Check sheet for the modelled part. Datum: model origin and axes. Units: mm. Face numbers are marked on the shaded views. Round coordinates to 2 decimals unless told otherwise and drop trailing zeros.
Item 1: Go/stop test with flat-tipped pins: pin 1 Ø0.9 at (y, z) = (47.5, 2) entering from -X; pin 2 Ø5.5 at (x, y) = (-15, -38.31) entering from +Z; pin 3 Ø6 at (x, y) = (-57, -19.5) entering from -Z; pin 4 Ø5 at (x, y) = (-17.5, 51.5) entering from +Z. Record where each tip stops, or that it passes through.
Item 2: Cross-section at A-A on y = -38.31. Count the separate pieces of the cut face and the enclosed holes in it, plus the area to 3 significant figures.
Item 3: Release check for a two-part mould opening along X. For the marked faces 1 and 2 record: +X half, -X half, draft (parallel to the pull), parting line (faces both ways), or undercut.
Item 4: Material ranges on line 1 (X direction, y = -38.31, z = 0.65); line 2 (X direction, y = -38.31, z = 0.75); line 3 (X direction, y = 30.5, z = 1.65), recorded low to high.
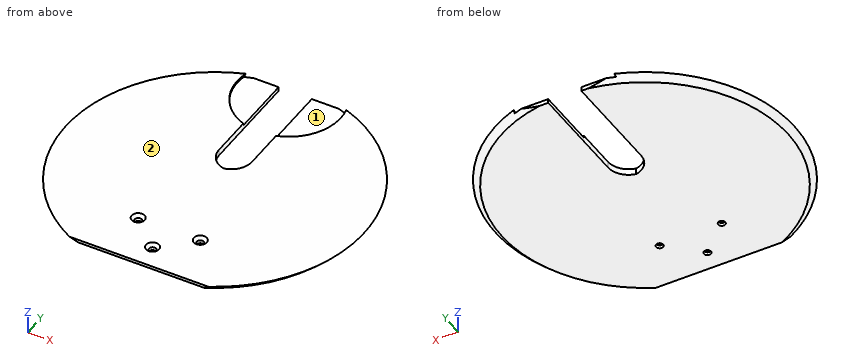
from build123d import *

# Parameters (mm, degrees)
BOSS_EXTRUDE2_DEPTH                                 = 3
CSK_FOR_M3_COUNTERSUNK_FLAT_HEAD_SCREW1_D           = 3.4
CSK_FOR_M3_COUNTERSUNK_FLAT_HEAD_SCREW1_DEPTH       = 3
CSK_FOR_M3_COUNTERSUNK_FLAT_HEAD_SCREW1_CSINK_D     = 6.3
CSK_FOR_M3_COUNTERSUNK_FLAT_HEAD_SCREW1_CSINK_ANGLE = 90
CSK_FOR_M3_COUNTERSUNK_FLAT_HEAD_SCREW1_TIP         = 1.021463052
SKETCH4_W                                           = 16
SKETCH4_H                                           = 60
CUT_EXTRUDE1_DEPTH                                  = 3
SKETCH5_R                                           = 25
CUT_EXTRUDE2_DEPTH                                  = 1
FILLET1_R                                           = 10
CUT_EXTRUDE3_DEPTH                                  = 21
CHAMFER2_SIZE                                       = 5
CHAMFER2_SIZE_2                                     = 2.886751346


with BuildPart() as part:
    # Sketch1 → Boss-Extrude2 (new body)
    with BuildSketch(Plane.XY):
        with BuildLine():
            Line((-23.664319132, 68), (23.664319132, 68))
            ThreePointArc((23.664319132, 68), (0, -72), (-23.664319132, 68))
        make_face()
    extrude(amount=BOSS_EXTRUDE2_DEPTH)

    # CSK for M3 Countersunk Flat Head Screw1
    with Locations(Plane.XY.offset(3)):
        with Locations((15, -38.31), (-15, -38.31), (0, -52.31)):
            CounterSinkHole(CSK_FOR_M3_COUNTERSUNK_FLAT_HEAD_SCREW1_D / 2, CSK_FOR_M3_COUNTERSUNK_FLAT_HEAD_SCREW1_CSINK_D / 2, depth=CSK_FOR_M3_COUNTERSUNK_FLAT_HEAD_SCREW1_DEPTH, counter_sink_angle=CSK_FOR_M3_COUNTERSUNK_FLAT_HEAD_SCREW1_CSINK_ANGLE)
            with Locations((0, 0, -(CSK_FOR_M3_COUNTERSUNK_FLAT_HEAD_SCREW1_DEPTH + CSK_FOR_M3_COUNTERSUNK_FLAT_HEAD_SCREW1_TIP / 2))):  # 118° drill point
                Cone(0, CSK_FOR_M3_COUNTERSUNK_FLAT_HEAD_SCREW1_D / 2, CSK_FOR_M3_COUNTERSUNK_FLAT_HEAD_SCREW1_TIP, mode=Mode.SUBTRACT)

    # Sketch4 → Cut-Extrude1 (cut)
    with BuildSketch(Plane.XY.offset(3)):
        with Locations((-0.5, 38)):
            Rectangle(SKETCH4_W, SKETCH4_H)
    extrude(amount=-CUT_EXTRUDE1_DEPTH, mode=Mode.SUBTRACT)

    # Sketch5 → Cut-Extrude2 (cut)
    with BuildSketch(Plane.XY.offset(3)):
        with Locations((0, 61.9)):
            Circle(SKETCH5_R)
    extrude(amount=-CUT_EXTRUDE2_DEPTH, mode=Mode.SUBTRACT)

    # Fillet1
    # the kernel refuses this fillet: 10 mm, written as the material it adds along each edge
    with BuildSketch(Plane(origin=(-8.5, 8, 3), x_dir=(1, 0, 0), z_dir=(0, 0, -1)), Plane(origin=(7.5, 8, 3), x_dir=(0, 1, 0), z_dir=(0, 0, -1))) as fillet1_piece_1:
        with BuildLine():
            CenterArc((FILLET1_R, -FILLET1_R), FILLET1_R, 90, 90)
            Line((0, -FILLET1_R), (0, 0))
            Line((0, 0), (FILLET1_R, 0))
        make_face()
    extrude(amount=3)

    # Sketch1<3> → Cut-Extrude3 (cut)
    with BuildSketch(Plane.XY):
        with BuildLine():
            Line((31.363416587, -64.81), (-31.363416587, -64.81))
            ThreePointArc((-31.363416587, -64.81), (0, -72), (31.363416587, -64.81))
        make_face()
    extrude(amount=CUT_EXTRUDE3_DEPTH, mode=Mode.SUBTRACT)

    # Chamfer2
    # the kernel refuses this chamfer: 5, 2.886751346 mm, written as the material it takes off along each edge
    with BuildSketch(Plane(origin=(44.29884536, -64.81, 0), x_dir=(0, -0.019326765612699606, 0.9998132206222079), z_dir=(-1, 0, 0))) as chamfer2_piece_1:
        Polygon((CHAMFER2_SIZE * 0.999813220622, CHAMFER2_SIZE * 0.0193267656127), (-CHAMFER2_SIZE_2 * 0.0193267656124, CHAMFER2_SIZE_2 * 0.999813220604), (0, 0), align=None)
    extrude(amount=88.59769072, mode=Mode.SUBTRACT)

    # Chamfer3
    # the kernel refuses this chamfer: 3 mm, written as the material it takes off along each edge
    with BuildSketch(Plane(origin=(0, 0, 0), x_dir=(0.07743421660335849, 0.9969974634366048, 0), z_dir=(-0.9969974634366048, 0.07743421660335849, 0))) as chamfer3_piece_1:
        with BuildLine():
            Line((72.084852814, -3.084852814), (68.915147186, 0.084852814))
            Line((68.915147186, 0.084852814), (68.915147186, 0.144852814))
            ThreePointArc((68.915147186, 0.144852814), (70.457573593, 0.06), (72, 0.06))
            Line((72, 0.06), (72.06, 0))
            ThreePointArc((72.06, 0), (72.06, -1.542426407), (72.144852814, -3.084852814))
            Line((72.144852814, -3.084852814), (72.084852814, -3.084852814))
        make_face()
    revolve(axis=Axis((0, 0, 0), (0, 0, -1)), revolution_arc=159.627586722, mode=Mode.SUBTRACT)
    with BuildSketch(Plane(origin=(0, 0, 0), x_dir=(-0.27448479603236836, -0.9615914396182347, 0), z_dir=(0.9615914396182347, -0.27448479603236836, 0))) as chamfer3_piece_2:
        with BuildLine():
            Line((72.084852814, -3.084852814), (68.915147186, 0.084852814))
            Line((68.915147186, 0.084852814), (68.915147186, 0.144852814))
            ThreePointArc((68.915147186, 0.144852814), (70.457573593, 0.06), (72, 0.06))
            Line((72, 0.06), (72.06, 0))
            ThreePointArc((72.06, 0), (72.06, -1.542426407), (72.144852814, -3.084852814))
            Line((72.144852814, -3.084852814), (72.084852814, -3.084852814))
        make_face()
    revolve(axis=Axis((0, 0, 0), (0, 0, -1)), revolution_arc=159.627586722, mode=Mode.SUBTRACT)


solid = part.part
Response values:
1. pin 1: stops at x = -53.49
1. pin 2: stops at z = 2.6
1. pin 3: stops at z = 0
1. pin 4: stops at z = 2
2. separate pieces: 3
2. enclosed holes: 0
2. area: 330 mm2
3. face 1: undercut
3. face 2: draft
4. line 1: x = -58.17 to -16.7, -13.3 to 13.3, 16.7 to 58.17
4. line 2: x = -58.29 to -16.7, -13.3 to 13.3, 16.7 to 58.29
4. line 3: x = -63.73 to -8.5, 7.5 to 63.73
